```python
from build123d import *

# Parameters (mm, degrees)
SKETCH1_W           = 10
SKETCH1_H           = 2.5
BOSS_EXTRUDE1_DEPTH = 2.5


with BuildPart() as part:
    # Sketch1 → Boss-Extrude1 (new body)
    with BuildSketch(Plane.XY):
        with BuildLine():
            Line((20, 0), (45, 0))
            ThreePointArc((45, 0), (50, -5), (55, 0))
            Line((55, 0), (95, 0))
            ThreePointArc((95, 0), (100, -5), (105, 0))
            Line((105, 0), (120, 0))
            Line((120, 0), (120, 10))
            Line((120, 10), (117.5, 10))
            Line((117.5, 10), (117.5, 20))
            Line((117.5, 20), (120, 20))
            Line((120, 20), (120, 30))
            Line((120, 30), (117.5, 30))
            Line((117.5, 30), (117.5, 40))
            Line((117.5, 40), (120, 40))
            Line((120, 40), (120, 50))
            Line((120, 50), (117.5, 50))
            Line((117.5, 50), (117.5, 60))
            Line((117.5, 60), (120, 60))
            Line((120, 60), (120, 70))
            Line((120, 70), (117.5, 70))
            Line((117.5, 70), (117.5, 80))
            Line((117.5, 80), (120, 80))
            Line((120, 80), (120, 90))
            Line((120, 90), (105, 90))
            ThreePointArc((105, 90), (100, 85), (95, 90))
            Line((95, 90), (55, 90))
            ThreePointArc((55, 90), (50, 85), (45, 90))
            Line((45, 90), (20, 90))
            Line((20, 90), (0, 45))
            Line((0, 45), (0, 40))
            Line((0, 40), (2.5, 40))
            Line((2.5, 40), (2.5, 35))
            Line((2.5, 35), (0, 35))
            Line((0, 35), (0, 30))
            Line((0, 30), (2.5, 30))
            Line((2.5, 30), (2.5, 25))
            Line((2.5, 25), (0, 25))
            Line((0, 25), (0, 15))
            Line((0, 15), (4, 12))
            Line((4, 12), (5.5, 14))
            Line((5.5, 14), (9.5, 11))
            Line((9.5, 11), (8, 9))
            Line((8, 9), (12, 6))
            Line((12, 6), (13.5, 8))
            Line((13.5, 8), (17.5, 5))
            Line((17.5, 5), (16, 3))
            Line((16, 3), (20, 0))
        make_face()
        with Locations((112.5, 3.75)):
            Rectangle(SKETCH1_W, SKETCH1_H, mode=Mode.SUBTRACT)
        with Locations((85, 3.75)):
            Rectangle(SKETCH1_W, SKETCH1_H, mode=Mode.SUBTRACT)
        with Locations((65, 3.75)):
            Rectangle(SKETCH1_W, SKETCH1_H, mode=Mode.SUBTRACT)
        with Locations((35, 3.75)):
            Rectangle(SKETCH1_W, SKETCH1_H, mode=Mode.SUBTRACT)
    extrude(amount=BOSS_EXTRUDE1_DEPTH)


solid = part.part
```
Model file for the job. Use its own axes, mm. A direction names the side the tool comes from. Coordinates: 2 decimals unless noted, no trailing zeros. Order: outer loops, then holes, each group sorted by start corner. A loop starts at its lowest first (then second) coordinate and runs counter-clockwise, first axis right, second up. Notation, with made-up numbers: (27.25, -9) -> (50.25, -9) arc R11 cw to (50.25, 7) -> close; hole circle Ø1 at (31.25, 64.25). An arc over 180 degrees is marked (long way). Return JSON: item names as keys, results as strings.
Item 1: 3-axis set-ups, long thin cutter, end or side, ignore diameter. For faces 5 (the face through (35, 5, 1)), 6 (the face through (119, 20, 1)), 7 (the face through (75, 0, 1)): which of +Z, -Z, +X, -X, +Y, -Y reach the whole face in a straight line?
Model answer:
{"face 5": "+Z, -Z", "face 6": "+Z, -Z, +X", "face 7": "+Z, -Z, -Y"}
Item 2: Pin check, flat tips, straight feed: P1, Ø1.2, axis at x = 119, z = 1, coming from the -Y side; P2, Ø0.8, axis at y = 3, z = 2, coming from the -X side; P3, Ø1.2, axis at x = 1.5, z = 1.5, coming from the -Y side (3 decimals). Stop position of each tip, or through.
Model answer:
{"P1": "stops at y = 0", "P2": "stops at x = 16", "P3": "stops at y = 13.425"}
Item 3: Slice it at A-A (x = 88). Write the cut outline in (y, z), then the cut area to 3 significant figures.
Model answer:
{"outline": "(0, 0) -> (2.5, 0) -> (2.5, 2.5) -> (0, 2.5) -> close; (5, 0) -> (90, 0) -> (90, 2.5) -> (5, 2.5) -> close", "area": "219 mm²"}
Item 4: Mould opens along Y. For faces 1 (the face through (100, -5, 1)), 2 (the face through (2.5, 38, 1)), 3 (the face through (10.14, 67.815, 1.232)), 4 (the face through (90, 4, 1)) say: pulls with the +Y half, pulls with the -Y half, needs draft (parallel to the pull), parting line crosses it, or undercut.
Model answer:
{"face 1": "pulls with the -Y half", "face 2": "undercut", "face 3": "pulls with the +Y half", "face 4": "undercut"}
Item 5: Wall check: line 1 along Y through (x, z) = (81, 1.9); line 2 along X through (y, z) = (4, 1.8); line 3 along X through (y, z) = (36.5, 1.15). Give the ranges that are in metal, low to high. Write a range as from..to.
Model answer:
{"line 1": "y = 0..2.5, 5..90", "line 2": "x = 16.75..30, 40..60, 70..80, 90..107.5, 117.5..120", "line 3": "x = 2.5..117.5"}
Item 6: Slice it at B-B (z = 1.5). Count the separate pieces of the cut face and the enclosed holes in it, then the cut area to 3 significant figures.
Model answer:
{"separate pieces": "1", "enclosed holes": "4", "area": "9,950 mm²"}
